The drawing under review shows one solid part. Ordinate dimensions are in mm from its lowest x, y, z. A direction names the side the tool comes from. Give positions to 0.01 mm unless a question says otherwise; leave off trailing zeros. Loops run counter-clockwise (first coordinate to the right, second up) from the corner with the lowest first, then second, coordinate; pieces in that order, holes last.
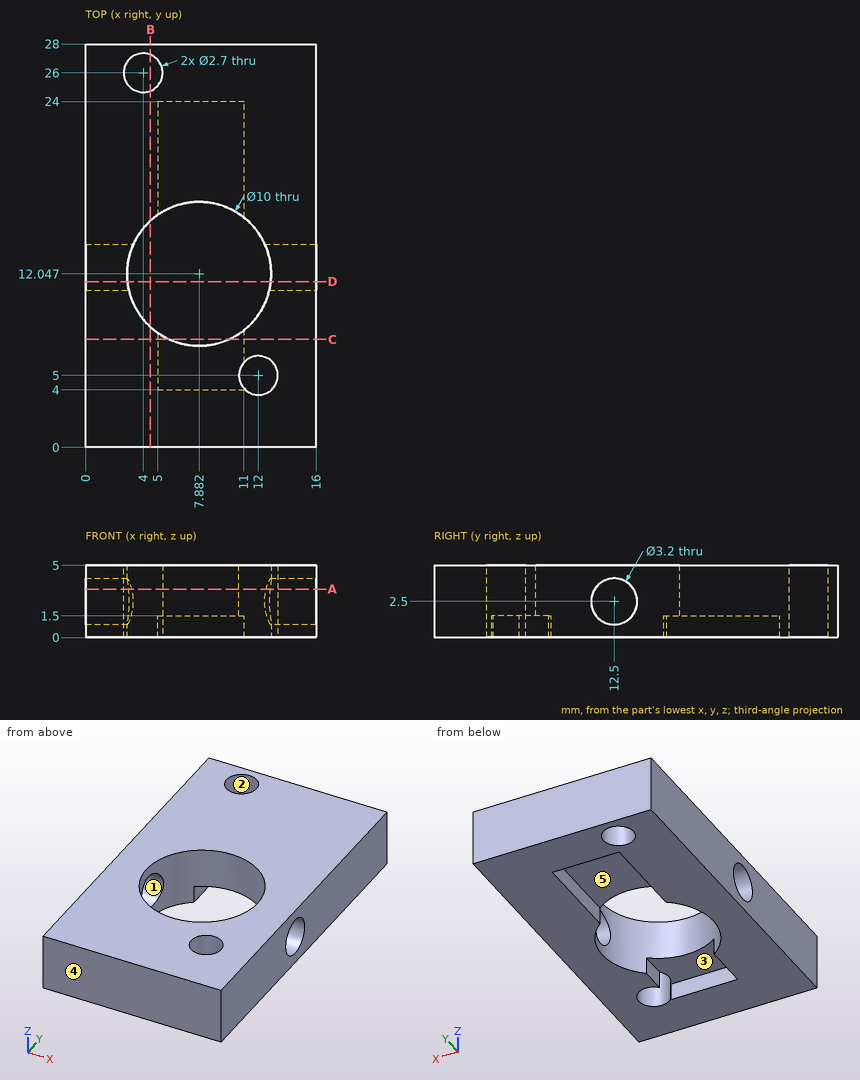
Item 1: Take a section at B-B on x = 4.5. Give the boundary of the cut face in (y, z) (1 decimal).
Answer:
outline: (0, 0) - (8.4, 0) - (8.4, 5) - (0, 5) - close; (15.7, 0) - (24.7, 0) - (24.7, 5) - (15.7, 5) - close; (27.3, 0) - (28, 0) - (28, 5) - (27.3, 5) - close
Item 2: Tool access review of the marked faces 4 and 5: name each direction out of +Z, -Z, +X, -X, +Y, -Y from which nothing blocks a thin tool from reaching the whole face with its end or side.
Answer:
face 4: +Z, -Z, +X, -X, -Y
face 5: -Z
Item 3: Take a section at C-C on y = 7.5. Give the boundary of the cut face in (x, z).
Answer:
outline: (0, 0) - (5, 0) - (5, 1.5) - (5.8, 1.5) - (5.8, 5) - (0, 5) - close; (9.96, 1.5) - (11, 1.5) - (11, 0) - (16, 0) - (16, 5) - (9.96, 5) - close
Item 4: Take a section at D-D on y = 11.5. Give the boundary of the cut face in (x, z).
Answer:
outline: (0, 0) - (2.91, 0) - (2.91, 1.25) - (0, 1.25) - close; (0, 3.75) - (2.91, 3.75) - (2.91, 5) - (0, 5) - close; (12.85, 0) - (16, 0) - (16, 1.25) - (12.85, 1.25) - close; (12.85, 3.75) - (16, 3.75) - (16, 5) - (12.85, 5) - close
Item 5: Take a section at A-A on z = 3.35. State how many separate pieces and enclosed holes the cut face has, and give its area (3 significant figures).
Answer:
separate pieces: 2
enclosed holes: 2
area: 341 mm2
Item 6: For L1, parallel to Z at x = 1.6, y = 12.5; L2, parallel to Y at x = 2.15, z = 2.5; L3, parallel to X at y = 5, z = 2.3, list the stretches that pass through material, from the lowest coordinate up.
Answer:
L1: z = 0 to 0.9, 4.1 to 5
L2: y = 0 to 10.9, 14.1 to 28
L3: x = 0 to 10.65, 13.35 to 16
Item 7: The part is to be moulded in two halves that separate along Z. For the marked faces 1, 2 and 3, say which applies: released by +Z, released by -Z, zero draft, split by the parting line, or undercut.
Answer:
face 1: undercut
face 2: zero draft
face 3: released by -Z
